Autodesk Inventor part; units mm, degrees
ref_plane "YZ Plane" through (0, 0, 0) normal (1, 0, 0) x (0, 1, 0)
ref_plane "XZ Plane" through (0, 0, 0) normal (0, 1, 0) x (-1, 0, 0)
ref_plane "XY Plane" through (0, 0, 0) normal (0, 0, 1) x (1, 0, 0)
sketch "Sketch1" plane through (0, 0, 0) normal (0, 0, 1) x (1, 0, 0)
  line L0 (0, 0) -> (31.75, 0)
  line L1 (31.75, 0) -> (31.75, 31.75)
  line L2 (31.75, 31.75) -> (0, 31.75)
  line L3 (0, 31.75) -> (0, 0)
  line L4 (0, 0) -> (0, 31.75)
  line L5 (0, 20.875) -> (-10, 20.875)
  line L6 (-10, 20.875) -> (-10, 10.875)
  line L7 (-10, 10.875) -> (0, 10.875)
  line L8 (0, 10.875) -> (0, 20.875)
  circle A0 centre (-5, 20.875) radius 2
  circle A1 centre (-5, 10.875) radius 2
  point P0 (-10, 15.875)
  point P1 (0, 15.875)
  point P2 (-7, 10.875)
  point P3 (-3, 10.875)
  point P4 (-3, 20.875)
  point P5 (-7, 20.875)
  dimension "d0" = 31.75
  dimension "d1" = 31.75
  dimension "d19" = 10
  dimension "d20" = 4
  dimension "d21" = 4
  dimension "d22" = 10
  dimension "d23" = 0
extrude "Extrusion1" add sketch "Sketch1" against normal blind 3.15 contours L3 L2 L1 L0 | L7 A1 L6 L5 A0 L3
sketch "Sketch2" plane through (0, 0, -3.15) normal (0, 0, -1) x (-1, 0, 0)
  circle A0 centre (-28.575, 28.575) radius 1.632
  circle A1 centre (-28.575, 28.575) radius 3
  line L0 (-28.575, 28.575) -> (-3.175, 28.575) construction
  line L1 (-3.175, 28.575) -> (-3.175, 3.175) construction
  line L2 (-3.175, 3.175) -> (-28.575, 3.175) construction
  line L3 (-28.575, 3.175) -> (-28.575, 28.575) construction
  line L4 (-31.75, 31.75) -> (-31.75, 0)
  line L5 (0, 31.75) -> (-31.75, 31.75)
  line L6 (-25.575, 28.575) -> (-25.575, 31.75)
  line L7 (-28.575, 25.575) -> (-31.75, 25.575)
  line L8 (-15.875, 28.575) -> (-15.875, 3.175) construction
  line L9 (-3.175, 15.875) -> (-28.575, 15.875) construction
  line L10 (-25.575, 3.175) -> (-25.575, 0)
  circle A2 centre (-28.575, 3.175) radius 1.632
  circle A3 centre (-28.575, 3.175) radius 3
  line L11 (-28.575, 6.175) -> (-31.75, 6.175)
  line L12 (-3.175, 6.175) -> (0, 6.175)
  circle A4 centre (-3.175, 3.175) radius 1.632
  circle A5 centre (-3.175, 3.175) radius 3
  line L13 (-6.175, 3.175) -> (-6.175, 0)
  line L14 (-6.175, 28.575) -> (-6.175, 31.75)
  circle A6 centre (-3.175, 28.575) radius 1.632
  circle A7 centre (-3.175, 28.575) radius 3
  line L15 (-3.175, 25.575) -> (0, 25.575)
  line L16 (-31.75, 0) -> (0, 0)
  line L17 (0, 20.875) -> (0, 31.75)
  line L18 (0, 0) -> (0, 10.875)
  point P0 (-31.75, 15.875)
  point P1 (10, 31.75)
  point P2 (-15.875, 15.875)
  point P3 (-15.875, 15.875)
  point P4 (10, 0)
  dimension "d5" = 3.2639
  dimension "d6" = 6
  dimension "d7" = 25.4
  dimension "d8" = 25.4
  dimension "d9" = 3.175
  dimension "d10" = 3.175
  dimension "d13" = 360
extrude "Extrusion2" cut sketch "Sketch2" against normal blind 2
extrude "Extrusion3" cut sketch "Sketch2" against normal through all contours A0 | A2 | A4 | A6
sketch "Sketch3" plane through (0, 0, -3.15) normal (0, 0, -1) x (-1, 0, 0)
  line L0 (3.5, 20.875) -> (6.5, 20.875)
  line L1 (6.5, 20.875) -> (6.5, 10.875)
  line L2 (6.5, 10.875) -> (3.5, 10.875)
  line L3 (3.5, 10.875) -> (3.5, 20.875)
  line L4 (7, 10.875) -> (10, 10.875)
  point P0 (0, 0)
  point P1 (3, 20.875)
  point P2 (3, 10.875)
  dimension "d26" = 0.5
  dimension "d27" = 0.5
  dimension "d28" = 3
extrude "Extrusion4" cut sketch "Sketch3" against normal blind 1.5
fillet "Fillet1" radius 1 6 edges at (-5, 18.875, -1.65) (-3, 20.875, -1.575) (-7, 20.875, -1.575) (-5, 12.875, -1.65) (-7, 10.875, -1.575) (-3, 10.875, -1.575)
fillet "Fillet2" radius 2 2 edges at (-10, 20.875, -1.575) (-10, 10.875, -1.575)
properties part number "lna605_base"
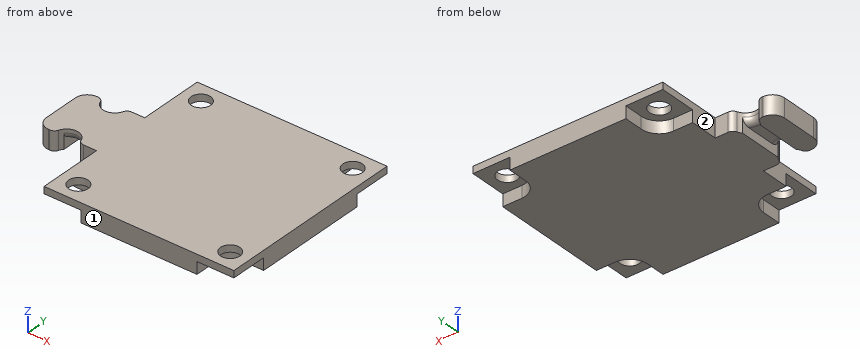
The listing builds one solid part. Answer for the finished solid, in the listing's coordinates (mm). Face numbers are marked on the shaded views. A direction names the side the tool comes from. Give positions to 0.01 mm unless a question says otherwise; leave off trailing zeros. Write each loop counter-clockwise with the first axis right and the second up, starting at its lowest first coordinate (ties: lowest second). Pieces come first, ordered by that corner, then holes. Notation, with made-up numbers: (85.25, 60) - (89.25, 60) arc R17 cw to (89.25, 84) - close; hole circle Ø10 at (83, -29). An arc over 180 degrees is marked (long way). Use one line per item in the form item = value. Start each with the question number.
1) Find section C-C on x = 29.5. Determine the outline of the cut face in (y, z) (3 decimals).
2) Flat-ended cylindrical pins translate along their axes: pin 1 Ø2.5 at (x, y) = (-5.5, 16) entering from -Z; pin 2 Ø1 at (y, z) = (22.5, -1) entering from -X; pin 3 Ø1.9 at (x, y) = (4.5, 3.5) entering from -Z; pin 4 Ø0.6 at (y, z) = (1.5, -2.5) entering from -X (3 decimals). Find the tip coordinate at first contact, or state that the pin passes through.
3) A tool of negligible diameter and unlimited length cuts with its end or side. For the marked faces 1 and 2, from which of +Z, -Z, +X, -X, +Y, -Y can it reach the whole face along a straight path? Write none if from no direction.
4) Consider line 1 along X through (y, z) = (16.5, -2.5); line 2 along X through (y, z) = (5, -0.2); line 3 along X through (y, z) = (28, -0.85). Determine where each line is inside the solid, lowest interval first. Write a range as from..to.
5) Find section B-B on y = 16.5. Determine the outline of the cut face in (x, z), plus the area to 3 significant figures.
6) Find section D-D on y = 26.5. Determine the outline of the cut face in (x, z), plus the area to 3 significant figures.
Geometry results:
q1.outline = (0, -1.15) - (1.83, -1.15) - (1.83, 0) - (0, 0) - close; (4.52, -1.15) - (6.175, -1.15) - (6.175, -3.15) - (25.575, -3.15) - (25.575, -1.15) - (27.23, -1.15) - (27.23, 0) - (4.52, 0) - close; (29.92, -1.15) - (31.75, -1.15) - (31.75, 0) - (29.92, 0) - close
q2.pin_1 = -3.15
q2.pin_2 = 0
q2.pin_3 = -1.15
q2.pin_4 = 6.175
q3.face_1 = +Z, -Z, +X, -X, -Y
q3.face_2 = +Z, -Z, -X, +Y
q4.line_1 = -10..-6.5, -3.5..31.75
q4.line_2 = 0..31.75
q4.line_3 = 0..1.65, 4.7..27.05, 30.1..31.75
q5.outline = (-10, -3.15) - (-6.5, -3.15) - (-6.5, -1.65) - (-3.5, -1.65) - (-3.5, -3.15) - (31.75, -3.15) - (31.75, 0) - (-10, 0) - close
q5.area = 127 mm2
q6.outline = (0, -1.15) - (5.34, -1.15) - (5.34, -3.15) - (26.41, -3.15) - (26.41, -1.15) - (31.75, -1.15) - (31.75, 0) - (0, 0) - close
q6.area = 78.6 mm2
